from build123d import *

# Parameters (mm, degrees)
SKETCH1_W               = 330
SKETCH1_H               = 167
BOSS_EXTRUDE1_DEPTH     = 2.5
SKETCH2_W               = 5
SKETCH2_H               = 15
BOSS_EXTRUDE2_DEPTH     = 10
SKETCH4_W               = 11
SKETCH4_H               = 5.2
CUT_EXTRUDE1_DEPTH      = 6
SKETCH5_W               = 4
SKETCH5_H               = 8
CUT_EXTRUDE2_DEPTH      = 6
MIRROR2_COPY_1_SKETCH_W = 5
MIRROR2_COPY_1_SKETCH_H = 15
MIRROR2_COPY_1_DEPTH    = 10
MIRROR2_COPY_2_SKETCH_W = 11
MIRROR2_COPY_2_SKETCH_H = 5.2
MIRROR2_COPY_2_DEPTH    = 6
MIRROR2_COPY_3_SKETCH_W = 4
MIRROR2_COPY_3_SKETCH_H = 8
MIRROR2_COPY_3_DEPTH    = 6


with BuildPart() as part:
    # Sketch1 → Boss-Extrude1 (new body, symmetric)
    with BuildSketch(Plane.XY):
        Rectangle(SKETCH1_W, SKETCH1_H)
    extrude(amount=BOSS_EXTRUDE1_DEPTH, both=True)

    # Sketch2 → Boss-Extrude2 (add)
    with BuildSketch(Plane.ZY.offset(165)):
        with Locations((0, 71)):
            Rectangle(SKETCH2_W, SKETCH2_H)
        with Locations((0, 41)):
            Rectangle(SKETCH2_W, SKETCH2_H)
    boss_extrude2 = extrude(amount=BOSS_EXTRUDE2_DEPTH)

    # Sketch4 → Cut-Extrude1 (cut, through all)
    with BuildSketch(Plane.XY.offset(2.5)):
        with Locations((-159.5, 56)):
            Rectangle(SKETCH4_W, SKETCH4_H)
    cut_extrude1 = extrude(amount=-CUT_EXTRUDE1_DEPTH, mode=Mode.SUBTRACT)

    # Sketch5 → Cut-Extrude2 (cut, through all)
    with BuildSketch(Plane.XY.offset(2.5)):
        with Locations((-159, 56)):
            Rectangle(SKETCH5_W, SKETCH5_H)
    cut_extrude2 = extrude(amount=-CUT_EXTRUDE2_DEPTH, mode=Mode.SUBTRACT)

    # Mirror1: Boss-Extrude2, Cut-Extrude1, Cut-Extrude2 across plane
    add(boss_extrude2.mirror(Plane.ZX))
    add(cut_extrude1.mirror(Plane.ZX), mode=Mode.SUBTRACT)
    add(cut_extrude2.mirror(Plane.ZX), mode=Mode.SUBTRACT)

    # Mirror2: Boss-Extrude2, Cut-Extrude1, Cut-Extrude2 across plane
    add(boss_extrude2.mirror(Plane(origin=(0, 0, 0), x_dir=(0, 0, 1), z_dir=(1, 0, 0))))
    add(cut_extrude1.mirror(Plane(origin=(0, 0, 0), x_dir=(0, 0, 1), z_dir=(1, 0, 0))), mode=Mode.SUBTRACT)
    add(cut_extrude2.mirror(Plane(origin=(0, 0, 0), x_dir=(0, 0, 1), z_dir=(1, 0, 0))), mode=Mode.SUBTRACT)

    # Mirror2 copy 1 sketch → Mirror2 copy 1 (add)
    with BuildSketch(Plane(origin=(165, 0, 0), x_dir=(0, 0, 1), z_dir=(1, 0, 0))):
        with Locations((0, 71)):
            Rectangle(MIRROR2_COPY_1_SKETCH_W, MIRROR2_COPY_1_SKETCH_H)
        with Locations((0, 41)):
            Rectangle(MIRROR2_COPY_1_SKETCH_W, MIRROR2_COPY_1_SKETCH_H)
    extrude(amount=MIRROR2_COPY_1_DEPTH)

    # Mirror2 copy 2 sketch → Mirror2 copy 2 (cut, through all)
    with BuildSketch(Plane(origin=(0, 0, 2.5), x_dir=(-1, 0, 0), z_dir=(0, 0, 1))):
        with Locations((-159.5, 56)):
            Rectangle(MIRROR2_COPY_2_SKETCH_W, MIRROR2_COPY_2_SKETCH_H)
    extrude(amount=-MIRROR2_COPY_2_DEPTH, mode=Mode.SUBTRACT)

    # Mirror2 copy 3 sketch → Mirror2 copy 3 (cut, through all)
    with BuildSketch(Plane(origin=(0, 0, 2.5), x_dir=(-1, 0, 0), z_dir=(0, 0, 1))):
        with Locations((-159, 56)):
            Rectangle(MIRROR2_COPY_3_SKETCH_W, MIRROR2_COPY_3_SKETCH_H)
    extrude(amount=-MIRROR2_COPY_3_DEPTH, mode=Mode.SUBTRACT)


solid = part.part
Model file for the job. Use its own axes, mm. Coordinates: 2 decimals unless noted, no trailing zeros. Write each loop counter-clockwise with the first axis right and the second up, starting at its lowest first coordinate (ties: lowest second). Pieces come first, ordered by that corner, then holes. Notation, with made-up numbers: (-38.5, 88.5) -> (10.5, 88.5) arc R31 cw to (10.5, 124.5) -> close; hole circle Ø2 at (-24.5, 79.5). An arc over 180 degrees is marked (long way). One line per item, written item: value. Start each with the question number.
1) Slice it at A-A on y = -10.5. Write the cut outline in (x, z), then the cut area to 3 significant figures.
2) Probe probe 1 along Y at (x, z) = (158.5, -2.05); probe 2 along X at (y, z) = (-56.5, 0.3); probe 3 along X at (y, z) = (-26.5, 2.2). List the from-to ranges inside material, lowest first.
3) Flat gauge pins, fed straight in: pin 1 Ø2.5 at (x, z) = (-168, 0.5) entering from -Y; pin 2 Ø1.5 at (y, z) = (-8.5, 0) entering from +X; pin 3 Ø1.1 at (y, z) = (-59.5, 0.5) entering from -X. Where does each tip first touch, or does it go through?
Answers follow:
1. outline: (-165, -2.5) -> (165, -2.5) -> (165, 2.5) -> (-165, 2.5) -> close
1. area: 1,650 mm2
2. probe 1: -83.5 to -60, -52 to 52, 60 to 83.5
2. probe 2: -154 to 154
2. probe 3: -165 to 165
3. pin 1: y = -78.5
3. pin 2: x = 165
3. pin 3: x = -165
